Could you check a few things on this drawing? It's one solid part, dimensions in mm from its lowest x, y, z. A direction names the side the tool comes from. Give positions to 0.01 mm unless a question says otherwise; leave off trailing zeros. Loops run counter-clockwise (first coordinate to the right, second up) from the corner with the lowest first, then second, coordinate; pieces in that order, holes last.
Q1. I need wall thicknesses on probe 1 along Y at (x, z) = (30, 59.3); probe 2 along Y at (x, z) = (30, 59); probe 3 along Z at (x, y) = (33, 158.5). Which ranges of each line are inside material? Lowest first, please.
Q2. For the marked faces 1 and 2, which set-ups out of +Z, -Z, +X, -X, +Y, -Y let a thin tool reach every point of the face, with its end or its side?
Q3. Suppose I cut it at B-B (x = 30). List the corners of the cut face in (y, z) for me.
Q4. Suppose I cut it at C-C (y = 35). List the corners of the cut face in (x, z) for me, and give its area (3 significant figures).
Q5. Suppose I cut it at D-D (x = 17). List the corners of the cut face in (y, z) for me, and give its area (3 significant figures).
Q6. Suppose I cut it at A-A (y = 115). List the corners of the cut face in (x, z) for me, and give its area (3 significant figures).
Q7. I'm going to push flat-ended pins straight in: P1, Ø1, axis at y = 29, z = 34, coming from the +X side; P2, Ø5, axis at x = 49, y = 166, coming from the +Z side; P3, Ø14.5, axis at x = 30, y = 35, coming from the +Z side; P4, Ø1, axis at x = 9, y = 152.5, coming from the -Z side. Where does each tip first touch, or does it pass through?
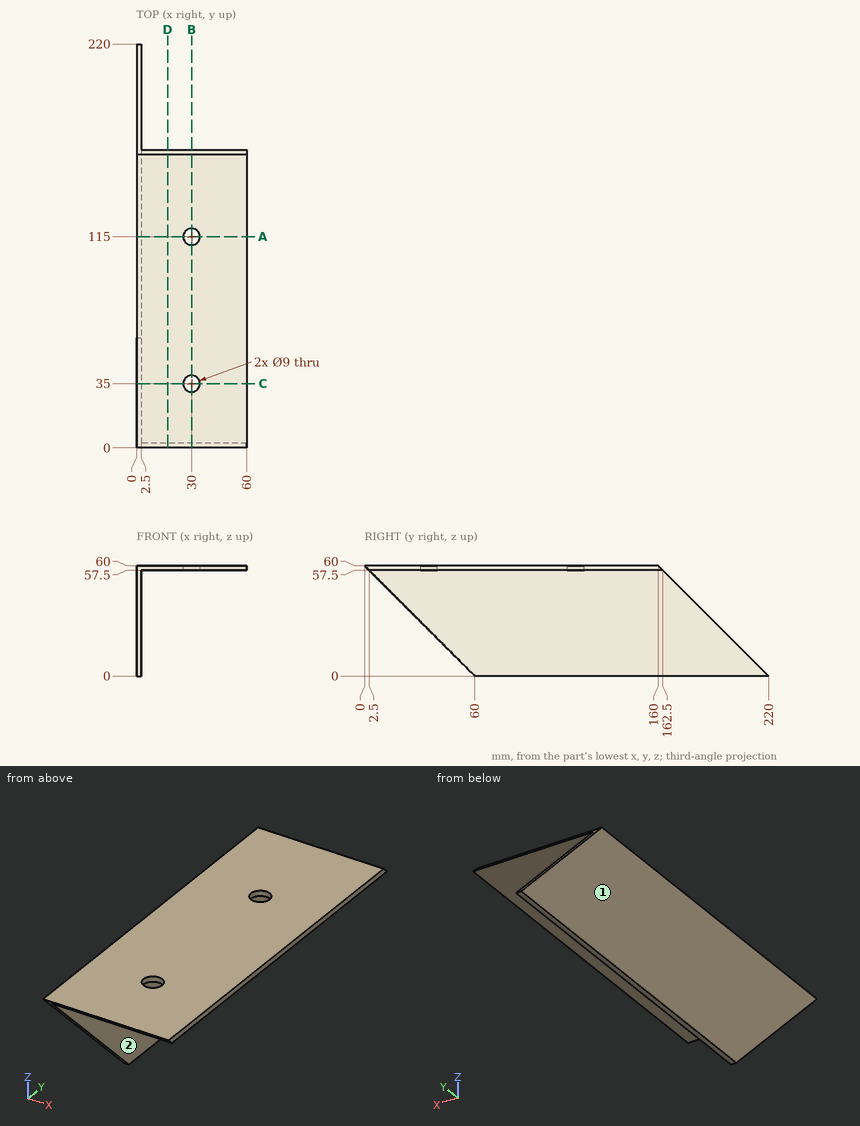
Solutions:
1. probe 1: y = 0.7 to 30.5, 39.5 to 110.5, 119.5 to 160.7
1. probe 2: y = 1 to 30.5, 39.5 to 110.5, 119.5 to 161
1. probe 3: z = 57.5 to 60
2. face 1: +Z, -Z, -X, +Y, -Y
2. face 2: -Z, +X, +Y, -Y
3. outline: (0, 60) - (2.5, 57.5) - (30.5, 57.5) - (30.5, 60) - close; (39.5, 57.5) - (110.5, 57.5) - (110.5, 60) - (39.5, 60) - close; (119.5, 57.5) - (162.5, 57.5) - (160, 60) - (119.5, 60) - close
4. outline: (0, 25) - (2.5, 25) - (2.5, 57.5) - (25.5, 57.5) - (25.5, 60) - (0, 60) - close; (34.5, 57.5) - (60, 57.5) - (60, 60) - (34.5, 60) - close
4. area: 209 mm2
5. outline: (0, 60) - (2.5, 57.5) - (162.5, 57.5) - (160, 60) - close
5. area: 400 mm2
6. outline: (0, 0) - (2.5, 0) - (2.5, 57.5) - (25.5, 57.5) - (25.5, 60) - (0, 60) - close; (34.5, 57.5) - (60, 57.5) - (60, 60) - (34.5, 60) - close
6. area: 271 mm2
7. P1: stops at x = 2.5
7. P2: passes through
7. P3: stops at z = 60
7. P4: stops at z = 57.5
